```python
from build123d import *

# Parameters (mm, degrees)
F0_R     = 6
F1_DEPTH = 100
F2_W     = 15
F2_H     = 100
F3_DEPTH = 5
F4_W     = 15
F4_H     = 100
F5_DEPTH = 5


with BuildPart() as f1:
    # F0 (on Top) → F1 (new body)
    with BuildSketch(Plane.XY):
        Circle(F0_R)
    extrude(amount=F1_DEPTH)

    # F2 (on Front) → F3 (join, symmetric)
    with BuildSketch(Plane.XZ):
        with Locations((-12.527533, 50)):
            Rectangle(F2_W, F2_H)
    extrude(amount=F3_DEPTH, both=True)

    # F4 (on Front) → F5 (join, symmetric)
    with BuildSketch(Plane.XZ):
        with Locations((13.012821, 50)):
            Rectangle(F4_W, F4_H)
    extrude(amount=F5_DEPTH, both=True)


solid = f1.part
```
Here's how the part is built. I have some questions about the finished solid (model axes, mm). A direction names the side the tool comes from. Coordinates: 2 decimals unless noted, no trailing zeros. Write each loop counter-clockwise with the first axis right and the second up, starting at its lowest first coordinate (ties: lowest second). Pieces come first, ordered by that corner, then holes. Notation, with made-up numbers: (19, -3.75) -> (47, -3.75) arc R28 ccw to (47, 17.25) -> close; hole circle Ø3 at (-33, 47.25). An arc over 180 degrees is marked (long way). Use a Markdown table: item, result. Add a question column.
(1) For faces 4 (the flat face through (-13, 5, 51)), 5 (the flat face through (13, 5, 51)), 6 (the flat face through (13, -5, 51)), 7 (the flat face through (-13, -5, 51)), which set-ups out of +Z, -Z, +X, -X, +Y, -Y let a thin tool reach every point of the face, with its end or its side?
(2) We'd pull the mould along X, two halves only. Please class faces 1 (the flat face through (-20.028, 0, 49)), 2 (the flat face through (0, 0, 0)), 3 (the flat face through (-5.028, -4, 49)): +X half, -X half, draft (parallel to the pull), parting line (faces both ways), or undercut.
(3) I'm going to push flat-ended pins straight in: P1, Ø4.5, axis at x = -16, z = 32, coming from the -Y side; P2, Ø4.5, axis at x = 16.5, z = 27, coming from the +Y side. Where does each tip first touch, or does it pass through?
(4) Please list where these lines run through material, in increasing order: line 1 (X direction, y = -4.75, z = 58); line 2 (Y direction, x = -13.5, z = 27); line 3 (X direction, y = 4, z = 78).
(5) If we section it at A-A, the plane z = 23.5: Write out the boundary of the cut face in (x, y), and give its area (3 significant figures).
(6) If we section it at B-B, the plane x = -6: Write out the boundary of the cut face in (y, z), and give its area (3 significant figures).
Outcome:
| question | item | result |
|---|---|---|
| 1 | face 4 | +Z, -Z, -X, +Y |
| 1 | face 5 | +Z, -Z, +X, +Y |
| 1 | face 6 | +Z, -Z, +X, -Y |
| 1 | face 7 | +Z, -Z, -X, -Y |
| 2 | face 1 | -X half |
| 2 | face 2 | draft |
| 2 | face 3 | undercut |
| 3 | P1 | stops at y = -5 |
| 3 | P2 | stops at y = 5 |
| 4 | line 1 | x = -20.03 to -5.03, -3.67 to 3.67, 5.51 to 20.51 |
| 4 | line 2 | y = -5 to 5 |
| 4 | line 3 | x = -20.03 to -5.03, -4.47 to 4.47, 5.51 to 20.51 |
| 5 | outline | (-20.03, -5) -> (-5.03, -5) -> (-5.03, -3.27) arc R6 ccw to (5.51, -2.37) -> (5.51, -5) -> (20.51, -5) -> (20.51, 5) -> (5.51, 5) -> (5.51, 2.37) arc R6 ccw to (-5.03, 3.27) -> (-5.03, 5) -> (-20.03, 5) -> close |
| 5 | area | 407 mm^2 |
| 6 | outline | (-5, 0) -> (5, 0) -> (5, 100) -> (-5, 100) -> close |
| 6 | area | 1,000 mm^2 |
